Check sheet for the modelled part. Datum: model origin and axes. Units: mm. Coordinates: 2 decimals unless noted, no trailing zeros. Loops run counter-clockwise (first coordinate to the right, second up) from the corner with the lowest first, then second, coordinate; pieces in that order, holes last. Notation, with made-up numbers: (-36, 25) -> (-16, 25) arc R12 cw to (-16, 32) -> close; hole circle Ø6 at (-14, 39.25). An arc over 180 degrees is marked (long way). Use one line per item in the form item = value.
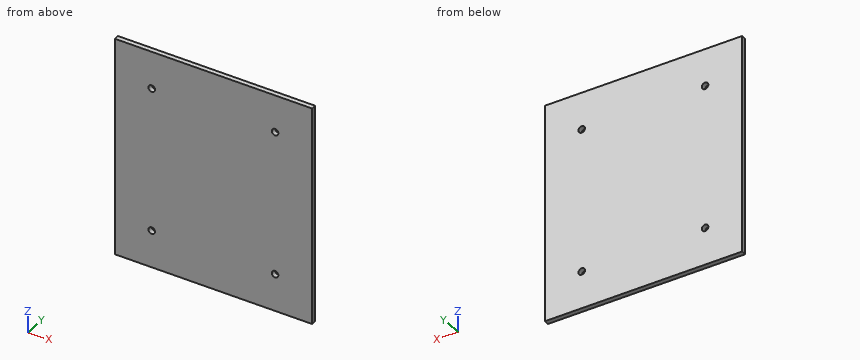
from build123d import *

# Parameters (mm, degrees)
SKETCH2_W           = 120
SKETCH2_H           = 132
SKETCH2_W_2         = 95
SKETCH2_H_2         = 107
SKETCH2_R           = 2
BOSS_EXTRUDE1_DEPTH = 3


with BuildPart() as part:
    # Sketch2 → Boss-Extrude1 (new body)
    # profile 1 of 3: a face of its own
    with BuildSketch(Plane(origin=(0, 0, 0), x_dir=(1, 0, 0), z_dir=(0, 1, 0))):
        Rectangle(SKETCH2_W, SKETCH2_H)
        Rectangle(SKETCH2_W_2, SKETCH2_H_2, mode=Mode.SUBTRACT)
    # profile 2 of 3: a face of its own
    with BuildSketch(Plane(origin=(0, 0, 0), x_dir=(1, 0, 0), z_dir=(0, 1, 0))):
        with BuildLine():
            ThreePointArc((37.5, -45.5), (36.085786438, -42.085786438), (39.5, -43.5))
            Line((39.5, -43.5), (47.5, -43.5))
            Line((47.5, -43.5), (47.5, 53.5))
            Line((47.5, 53.5), (-47.5, 53.5))
            Line((-47.5, 53.5), (-47.5, -53.5))
            Line((-47.5, -53.5), (37.5, -53.5))
            Line((37.5, -53.5), (37.5, -45.5))
        make_face()
        with Locations(Location((-37.5, -43.5, 0), (0, 0, 270))):
            Circle(SKETCH2_R, mode=Mode.SUBTRACT)
        with Locations(Location((-37.5, 43.5, 0), (0, 0, 270))):
            Circle(SKETCH2_R, mode=Mode.SUBTRACT)
        with Locations(Location((37.5, 43.5, 0), (0, 0, 270))):
            Circle(SKETCH2_R, mode=Mode.SUBTRACT)
    # profile 3 of 3: a face of its own
    with BuildSketch(Plane(origin=(0, 0, 0), x_dir=(1, 0, 0), z_dir=(0, 1, 0))):
        with BuildLine():
            Line((47.5, -43.5), (39.5, -43.5))
            ThreePointArc((39.5, -43.5), (38.914213562, -44.914213562), (37.5, -45.5))
            Line((37.5, -45.5), (37.5, -53.5))
            Line((37.5, -53.5), (47.5, -53.5))
            Line((47.5, -53.5), (47.5, -43.5))
        make_face()
    extrude(amount=BOSS_EXTRUDE1_DEPTH)


solid = part.part
(1) Section check A-A, the plane x = -37.5. Record the boundary of the cut face in (y, z).
Established:
outline = (0, -66) -> (3, -66) -> (3, -45.5) -> (0, -45.5) -> close; (0, -41.5) -> (3, -41.5) -> (3, 41.5) -> (0, 41.5) -> close; (0, 45.5) -> (3, 45.5) -> (3, 66) -> (0, 66) -> close
(2) Section check B-B, the plane z = -43.5. Record the boundary of the cut face in (x, y).
Established:
outline = (-60, 0) -> (-39.5, 0) -> (-39.5, 3) -> (-60, 3) -> close; (-35.5, 0) -> (35.5, 0) -> (35.5, 3) -> (-35.5, 3) -> close; (39.5, 0) -> (60, 0) -> (60, 3) -> (39.5, 3) -> close
(3) Go/stop test with flat-tipped pins: P1, Ø4.5, axis at x = 37.5, z = -43.5, coming from the +Y side; P2, Ø3.5, axis at x = -37.5, z = 43.5, coming from the +Y side. Record where each tip stops, or that it passes through.
Established:
P1 = 3
P2 = through
(4) Scan line: line 1 along X through (y, z) = (1.25, 43.5). Record every from-to range of solid material in increasing order.
Established:
line_1 = -60 to -39.5, -35.5 to 35.5, 39.5 to 60
